For this review, take the finished solid that the model builds, in its own axes (mm). A direction names the side the tool comes from. Give positions to 0.01 mm unless a question says otherwise; leave off trailing zeros. Write each loop counter-clockwise with the first axis right and the second up, starting at its lowest first coordinate (ties: lowest second). Pieces come first, ordered by that corner, then holes.
Q1. Machinability: for faces 1 (the flat face through (100, 306, -139)), 2 (the flat face through (-100, 306, -139)), 3 (the flat face through (1.4, 294.65, -130.73)), which of the approach directions +Z, -Z, +X, -X, +Y, -Y give a long, thin tool a straight path to every point of the face, cutting with its end or side? Answer none if there is none.
Q2. For line 1 (Z direction, x = -78.5, y = 149); line 2 (Z direction, x = -342.5, y = 83.5); line 3 (X direction, y = -105.5, z = 22), list the stretches that pass through material, from the lowest coordinate up.
Q3. We need section A-A (y = 282.5). Write out the cut boundary in (x, z).
Q4. We need section D-D (z = -120.5). Write out the cut boundary in (x, y), then the cut area to 3 significant figures.
Q5. We need section B-B (x = -15). Write out the cut boundary in (y, z).
Q6. Insertion check: P1, Ø12, axis at x = -27, z = -176, coming from the +Y side; P2, Ø8, axis at x = 140.5, y = -124, coming from the -Z side; P3, Ø1.5, axis at x = -83, y = 288.5, coming from the +Z side. Each pin has a flat end and moves straight along its axis. Give the tip position at first contact, or say it passes through.
Q7. We need section C-C (y = -271). Write out the cut boundary in (x, z).
```python
from build123d import *

# Parameters (mm, degrees)
F1_DEPTH = 10
F2_W     = 887.253195621
F2_H     = 100
F3_DEPTH = 10
F6_DEPTH = 100


with BuildPart() as f1:
    # F0 (on Top) → F1 (new body)
    with BuildSketch(Plane.XY):
        Polygon((-300, -442.5), (300, -442.5), (375, 442.5), (300, 442.5), (-300, 442.5), (-375, 442.5), align=None)
    extrude(amount=F1_DEPTH)

    # F2 (on face) → F3 (join)
    with BuildSketch(Plane(origin=(-335.0934112949, -28.3977467199, 0), x_dir=(0.0844430767, -0.9964283049, 0), z_dir=(-0.9964283049, -0.0844430767, 0))):
        with Locations((-28.9590808637, 50)):
            Rectangle(F2_W, F2_H)
    extrude(amount=-F3_DEPTH)

    # F4: F1 across plane


with BuildPart() as f1_1:
    add(f1.part)
    add(f1.part.mirror(Plane.YZ))

    # F5 (on Right) → F6 (join, symmetric)
    with BuildSketch(Plane.YZ):
        Polygon((185.2948494855, -278.7305519032), (442.5, 0), (415.2859534537, 0), (170.5965575825, -265.1673585059), align=None)
    extrude(amount=F6_DEPTH, both=True)


solid = f1_1.part
```
Computed:
1. face 1: -Z, +X, +Y, -Y
1. face 2: -Z, -X, +Y, -Y
1. face 3: +X, -X, -Y
2. line 1: z = 0 to 10
2. line 2: z = 0 to 100
2. line 3: x = -328.56 to -318.52, 318.52 to 328.56
3. outline: (-361.44, 0) - (361.44, 0) - (361.44, 100) - (351.4, 100) - (351.4, 10) - (-351.4, 10) - (-351.4, 100) - (-361.44, 100) - close; (-100, -173.39) - (100, -173.39) - (100, -143.9) - (-100, -143.9) - close
4. outline: (-100, 304.09) - (100, 304.09) - (100, 331.31) - (-100, 331.31) - close
4. area: 5,440 mm2
5. outline: (-442.5, 0) - (415.29, 0) - (170.6, -265.17) - (185.29, -278.73) - (442.5, 0) - (442.5, 10) - (-442.5, 10) - close
6. P1: stops at y = 285.63
6. P2: stops at z = 0
6. P3: stops at z = 10
7. outline: (-314.53, 0) - (314.53, 0) - (314.53, 100) - (304.5, 100) - (304.5, 10) - (-304.5, 10) - (-304.5, 100) - (-314.53, 100) - close
